```python
from build123d import *

# Parameters (mm, degrees)
SCHIZZO1_R                   = 1
ESTRUSIONE_ESTRUSIONE1_DEPTH = 2
SMUSSO1_SIZE                 = 1.5


with BuildPart() as part:
    # Schizzo1 → Estrusione-Estrusione1 (new body)
    with BuildSketch(Plane.XY):
        with BuildLine():
            Line((-23, -18.5), (23, -18.5))
            ThreePointArc((23, -18.5), (25.828427125, -17.328427125), (27, -14.5))
            Line((27, -14.5), (28, -14.5))
            ThreePointArc((28, -14.5), (31.5, -11), (28, -7.5))
            Line((28, -7.5), (27, -7.5))
            Line((27, -7.5), (27, 7.5))
            Line((27, 7.5), (28, 7.5))
            ThreePointArc((28, 7.5), (31.5, 11), (28, 14.5))
            Line((28, 14.5), (27, 14.5))
            ThreePointArc((27, 14.5), (25.828427125, 17.328427125), (23, 18.5))
            Line((23, 18.5), (-23, 18.5))
            ThreePointArc((-23, 18.5), (-25.828427125, 17.328427125), (-27, 14.5))
            Line((-27, 14.5), (-28, 14.5))
            ThreePointArc((-28, 14.5), (-31.5, 11), (-28, 7.5))
            Line((-28, 7.5), (-27, 7.5))
            Line((-27, 7.5), (-27, -7.5))
            Line((-27, -7.5), (-28, -7.5))
            ThreePointArc((-28, -7.5), (-31.5, -11), (-28, -14.5))
            Line((-28, -14.5), (-27, -14.5))
            ThreePointArc((-27, -14.5), (-25.828427125, -17.328427125), (-23, -18.5))
        make_face()
        with Locations((-28, 11)):
            Circle(SCHIZZO1_R, mode=Mode.SUBTRACT)
        with Locations((-28, -11)):
            Circle(SCHIZZO1_R, mode=Mode.SUBTRACT)
        with Locations((28, -11)):
            Circle(SCHIZZO1_R, mode=Mode.SUBTRACT)
        with Locations((28, 11)):
            Circle(SCHIZZO1_R, mode=Mode.SUBTRACT)
    extrude(amount=ESTRUSIONE_ESTRUSIONE1_DEPTH)

    # Smusso1
    smusso1_edges = [part.edges().sort_by_distance(p)[0] for p in [
        (-29, 11, 2),
        (-29, -11, 2),
        (27, -11, 2),
        (27, 11, 2),
    ]]
    chamfer(smusso1_edges, length=SMUSSO1_SIZE)


solid = part.part
```
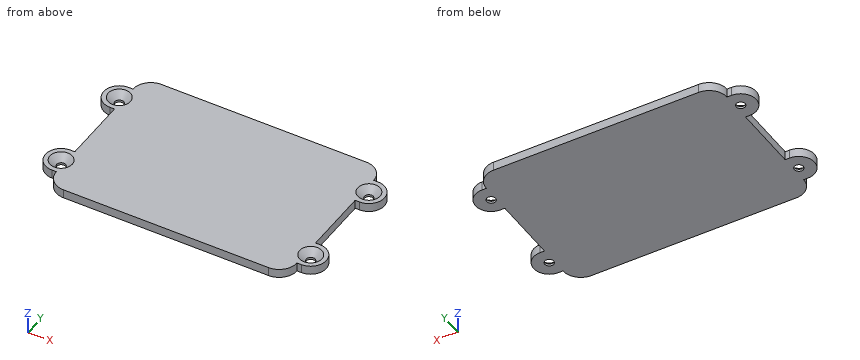
Input: part model. Units: mm. Frame: model coordinates. Round coordinates to 2 decimals unless told otherwise and drop trailing zeros. Loops run counter-clockwise (first coordinate to the right, second up) from the corner with the lowest first, then second, coordinate; pieces in that order, holes last. Notation, with made-up numbers: (59.5, -23) -> (80.5, -23) arc R23 ccw to (80.5, -4) -> close; hole circle Ø3 at (48.5, -14.75). An arc over 180 degrees is marked (long way). Use one line per item in the form item = value. Start each with the question number.
Item 1: Section query A-A on y = -11. Return the cut outline in (x, z).
Item 2: Contact query for flat-ended pins moving along their axis: pin 1 Ø2.5 at (x, y) = (-28, -11) entering from -Z; pin 2 Ø1 at (y, z) = (1.5, 1.5) entering from +X; pin 3 Ø0.5 at (x, z) = (27.5, 1) entering from +Y; pin 4 Ø0.8 at (x, z) = (27.5, 1.5) entering from -Y. Output: stop coordinate, or through.
Item 3: Section query C-C on y = -3. Return the cut outline in (x, z), then the cut area to 3 significant figures.
Item 4: Material intervals for L1, parallel to Y at x = 28, z = 0.15; L2, parallel to X at y = -6, z = 1.6; L3, parallel to X at y = -10.5, z = 1.95, sorted ascending. Write a range as from..to.
Item 5: Section query B-B on z = 1.3. Return the cut outline in (x, y), then the cut area to 3 significant figures.
Ans:
q1.outline = (-31.5, 0) -> (-29, 0) -> (-29, 0.5) -> (-30.5, 2) -> (-31.5, 2) -> close; (-27, 0) -> (27, 0) -> (27, 0.5) -> (25.5, 2) -> (-25.5, 2) -> (-27, 0.5) -> close; (29, 0) -> (31.5, 0) -> (31.5, 2) -> (30.5, 2) -> (29, 0.5) -> close
q2.pin_1 = 0
q2.pin_2 = 27
q2.pin_3 = 14.5
q2.pin_4 = -14.5
q3.outline = (-27, 0) -> (27, 0) -> (27, 2) -> (-27, 2) -> close
q3.area = 108 mm^2
q4.L1 = -14.5..-12, -10..-7.5, 7.5..10, 12..14.5
q4.L2 = -27..27
q4.L3 = -31.46..-30.4, -25.6..25.6, 30.4..31.46
q5.outline = (-28, -14.5) -> (-27, -14.5) arc R4 ccw to (-23, -18.5) -> (23, -18.5) arc R4 ccw to (27, -14.5) -> (28, -14.5) arc R3.5 ccw to (28, -7.5) -> (27, -7.5) -> (27, 7.5) -> (28, 7.5) arc R3.5 ccw to (28, 14.5) -> (27, 14.5) arc R4 ccw to (23, 18.5) -> (-23, 18.5) arc R4 ccw to (-27, 14.5) -> (-28, 14.5) arc R3.5 ccw to (-28, 7.5) -> (-27, 7.5) -> (-27, -7.5) -> (-28, -7.5) arc R3.5 ccw to start; hole circle Ø3.6 at (-28, -11); hole circle Ø3.6 at (-28, 11); hole circle Ø3.6 at (28, -11); hole circle Ø3.6 at (28, 11)
q5.area = 2,050 mm^2
